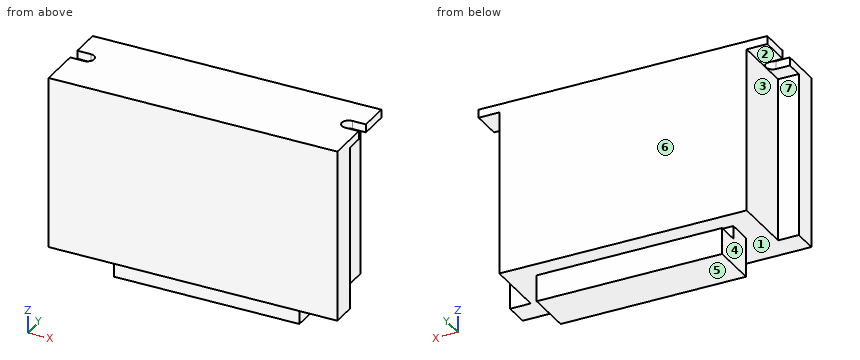
```python
from build123d import *

# Parameters (mm, degrees)
EXTRUDE_1_DEPTH     = 95
SKETCH_2_W          = 81.4
SKETCH_2_H          = 54.1
EXTRUDE_2_DEPTH     = 20
SKETCH_3_W          = 61
SKETCH_3_H          = 8
EXTRUDE_3_DEPTH     = 13
SKETCH_4_W          = 61
SKETCH_4_H          = 8.7
EXTRUDE_4_DEPTH     = 7.2
CUT_EXTRUDE_1_DEPTH = 70.8


with BuildPart() as part:
    # 草图1 → 凸台-拉伸1 (new body)
    with BuildSketch(Plane(origin=(0, 0, 0), x_dir=(0, 0, -1), z_dir=(1, 0, 0))):
        Polygon((0, 0), (-56.8, 0), (-56.8, 28), (-54.1, 28), (-54.1, 8), (0, 8), align=None)
    extrude(amount=EXTRUDE_1_DEPTH)

    # 草图2 → 凸台-拉伸2 (add)
    with BuildSketch(Plane(origin=(0, 8, 0), x_dir=(1, 0, 0), z_dir=(0, 1, 0))):
        with Locations((47.5, -27.05)):
            Rectangle(SKETCH_2_W, SKETCH_2_H)
    extrude(amount=EXTRUDE_2_DEPTH)

    # 草图3 → 凸台-拉伸3 (add)
    with BuildSketch(Plane(origin=(0, 0, 0), x_dir=(-1, 0, 0), z_dir=(0, 0, -1))):
        with Locations((-45, 17.553614205)):
            Rectangle(SKETCH_3_W, SKETCH_3_H)
    extrude(amount=EXTRUDE_3_DEPTH)

    # 草图4 → 凸台-拉伸4 (add)
    with BuildSketch(Plane(origin=(0, 21.553614205, 0), x_dir=(1, 0, 0), z_dir=(0, 1, 0))):
        with Locations((45, 8.65)):
            Rectangle(SKETCH_4_W, SKETCH_4_H)
    extrude(amount=EXTRUDE_4_DEPTH)

    # 草图7 → 切除-拉伸1 (cut, through all)
    with BuildSketch(Plane.XY.offset(56.8)):
        with BuildLine():
            Line((4.5, 18.2), (0, 18.2))
            Line((0, 18.2), (0, 13.7))
            Line((0, 13.7), (4.5, 13.7))
            ThreePointArc((4.5, 13.7), (6.75, 15.95), (4.5, 18.2))
        make_face()
        with BuildLine():
            Line((90.5, 13.7), (95, 13.7))
            Line((95, 13.7), (95, 18.2))
            Line((95, 18.2), (90.5, 18.2))
            ThreePointArc((90.5, 18.2), (88.25, 15.95), (90.5, 13.7))
        make_face()
    extrude(amount=-CUT_EXTRUDE_1_DEPTH, mode=Mode.SUBTRACT)


solid = part.part
```
Check sheet for the modelled part. Datum: model origin and axes. Units: mm. Face numbers are marked on the shaded views. A direction names the side the tool comes from. Give positions to 0.01 mm unless a question says otherwise; leave off trailing zeros. Order: outer loops, then holes, each group sorted by start corner. A loop starts at its lowest first (then second) coordinate and runs counter-clockwise, first axis right, second up. Notation, with made-up numbers: (-17, -26.5) -> (-8, -26.5) arc R21 cw to (-8, 1.5) -> close; hole circle Ø7 at (-14.5, 80.25). An arc over 180 degrees is marked (long way). Return JSON: item names as keys, results as strings.
1. Set-up check for the marked faces 4, 5, 6 and 7: record each of +Z, -Z, +X, -X, +Y, -Y from which the full face is reachable in a straight line by a thin tool's end or side.
From the geometry:
{"face 4": "-Z, -X, +Y, -Y", "face 5": "-Z, +X, -X, +Y, -Y", "face 6": "+Z, +X, -X, +Y", "face 7": "-Z, -X, +Y"}
2. Cross-section at D-D, the plane x = 58.5. Record the cut outline in (y, z), plus the area to 3 significant figures.
From the geometry:
{"outline": "(0, 0) -> (13.55, 0) -> (13.55, -13) -> (28.75, -13) -> (28.75, -4.3) -> (21.55, -4.3) -> (21.55, 0) -> (28, 0) -> (28, 56.8) -> (0, 56.8) -> close", "area": "1,760 mm^2"}
3. Mould release check, pull along Z, two halves, no side actions. Record for the marked faces 1, 2 and 3: +Z half, -Z half, draft (parallel to the pull), parting line (faces both ways), or undercut.
From the geometry:
{"face 1": "undercut", "face 2": "-Z half", "face 3": "draft"}
4. Material ranges on probe 1 along Z at (x, y) = (71, 22.75); probe 2 along Z at (x, y) = (85, 16); probe 3 along Z at (x, y) = (90.5, 21.5), recorded low to high. Write a range as [from, to].
From the geometry:
{"probe 1": "[-13, -4.3], [0, 56.8]", "probe 2": "[0, 56.8]", "probe 3": "[54.1, 56.8]"}
5. Cross-section at B-B, the plane y = 25.5. Record the cut outline in (x, z), plus the area to 3 significant figures.
From the geometry:
{"outline": "(0, 54.1) -> (6.8, 54.1) -> (6.8, 0) -> (88.2, 0) -> (88.2, 54.1) -> (95, 54.1) -> (95, 56.8) -> (0, 56.8) -> close; (14.5, -13) -> (75.5, -13) -> (75.5, -4.3) -> (14.5, -4.3) -> close", "area": "5,190 mm^2"}
6. Cross-section at A-A, the plane y = 11.25. Record the cut outline in (x, z), plus the area to 3 significant figures.
From the geometry:
{"outline": "(0, 54.1) -> (6.8, 54.1) -> (6.8, 0) -> (88.2, 0) -> (88.2, 54.1) -> (95, 54.1) -> (95, 56.8) -> (0, 56.8) -> close", "area": "4,660 mm^2"}
7. Cross-section at C-C, the plane z = 48. Record the cut outline in (x, y), plus the area to 3 significant figures.
From the geometry:
{"outline": "(0, 0) -> (95, 0) -> (95, 8) -> (88.2, 8) -> (88.2, 28) -> (6.8, 28) -> (6.8, 8) -> (0, 8) -> close", "area": "2,390 mm^2"}
8. Go/stop test with flat-tipped pins: P1, Ø1.5, axis at x = 63.5, y = 6.5, coming from the -Z side; P2, Ø8, axis at x = 33.5, z = 10, coming from the +Y side; P3, Ø6, axis at y = 17, z = 31.5, coming from the +X side. Record where each tip stops, or that it passes through.
From the geometry:
{"P1": "z = 0", "P2": "y = 28", "P3": "x = 88.2"}
